Part model, mm, in its own coordinate system. Face numbers are marked on the shaded views. Round coordinates to 2 decimals unless told otherwise and drop trailing zeros. Write each loop counter-clockwise with the first axis right and the second up, starting at its lowest first coordinate (ties: lowest second). Pieces come first, ordered by that corner, then holes.
from build123d import *

# Parameters (mm, degrees)
F0_R     = 84
F0_R_2   = 3
F1_DEPTH = 5
F2_SIZE  = 2
F3_SIZE  = 3


# Not quite as in the source:
# - a feature names something its author has since deleted; it is built from what else it names


with BuildPart() as f1:
    # F0 (on Front) → F1 (new body)
    with BuildSketch(Plane.XZ):
        Circle(F0_R)
        with Locations((-42.7799602618, -42.7799602618)):
            Circle(F0_R_2, mode=Mode.SUBTRACT)
        with Locations((42.7799602618, -42.7799602618)):
            Circle(F0_R_2, mode=Mode.SUBTRACT)
        with Locations((-42.7799602618, 42.7799602618)):
            Circle(F0_R_2, mode=Mode.SUBTRACT)
        with Locations((42.7799602618, 42.7799602618)):
            Circle(F0_R_2, mode=Mode.SUBTRACT)
    extrude(amount=F1_DEPTH)

    # F2
    f2_edges = [f1.edges().sort_by_distance(p)[0] for p in [
        (-84, -5, 0),
    ]]
    chamfer(f2_edges, length=F2_SIZE)

    # F3
    f3_edges = [f1.edges().sort_by_distance(p)[0] for p in [
        (-45.77996, -5, 42.77996),
        (39.77996, -5, 42.77996),
        (-45.77996, -5, -42.77996),
        (39.77996, -5, -42.77996),
    ]]
    chamfer(f3_edges, length=F3_SIZE)


solid = f1.part
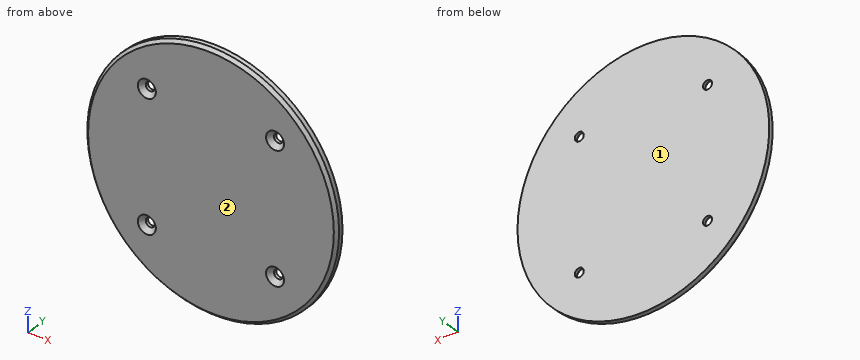
Q1. Two-plate mould, pull along Y, no slides. Class the marked faces 1 and 2: released by +Y, released by -Y, zero draft, split by the parting line, or undercut.
Q2. Wall check: line 1 (X direction, y = -1.5, z = -40.5); line 2 (X direction, y = -2.95, z = -46); line 3 (Z direction, x = 44.5, y = -2.05). Give the ranges that are in metal, low to high.
Q3. Drop flat-ended pins along their axis: P1, Ø5, axis at x = -42.78, z = 42.78, coming from the +Y side; P2, Ø3, axis at y = -3.5, z = -20.5, coming from the -X side; P3, Ø3, axis at x = -60.5, y = -3.5, coming from the -Z side; P4, Ø9.5, axis at x = -42.78, z = -42.78, coming from the -Y side. Give the stop position or say it passes through.
Q4. Saw through at A-A, the plane y = -1.15. Write the cut outline in (x, z), and give its area (3 significant figures).
Computed:
1. face 1: released by +Y
1. face 2: released by -Y
2. line 1: x = -73.59 to -44.73, -40.83 to 40.83, 44.73 to 73.59
2. line 2: x = -70.29 to -45.07, -40.49 to 40.49, 45.07 to 70.29
2. line 3: z = -71.24 to -45.3, -40.26 to 40.26, 45.3 to 71.24
3. P1: passes through
3. P2: stops at x = -81.8
3. P3: stops at z = -59.71
3. P4: stops at y = -3.75
4. outline: circle Ø168 at (0, 0); hole circle Ø6 at (-42.78, -42.78); hole circle Ø6 at (-42.78, 42.78); hole circle Ø6 at (42.78, -42.78); hole circle Ø6 at (42.78, 42.78)
4. area: 22,100 mm2
